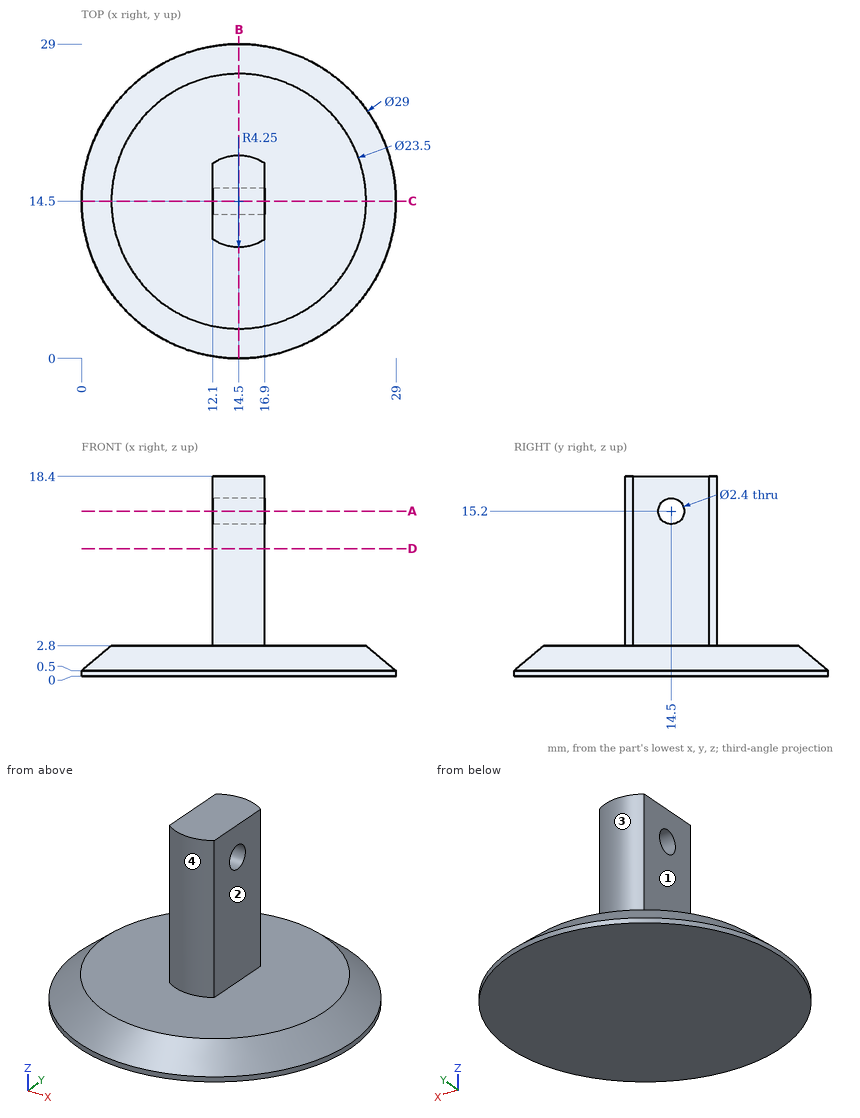
Study the drawing (mm; zero at the part's minimum x, y, z) and answer. A direction names the side the tool comes from. Round coordinates to 2 decimals unless told otherwise and drop trailing zeros. Loops run counter-clockwise (first coordinate to the right, second up) from the corner with the lowest first, then second, coordinate; pieces in that order, holes last. Notation, with made-up numbers: (-31, -1) -> (-6, -1) arc R7 ccw to (-6, 10) -> close; hole circle Ø11 at (18, 51). An arc over 180 degrees is marked (long way). Use one line per item in the form item = value.
1. A tool of negligible diameter and unlimited length cuts with its end or side. For the marked faces 1, 2, 3 and 4, from which of +Z, -Z, +X, -X, +Y, -Y can it reach the whole face along a straight path? Write none if from no direction.
Answer key:
face_1 = +Z, -X, +Y, -Y
face_2 = +Z, +X, +Y, -Y
face_3 = +Z, +Y
face_4 = +Z, -Y
2. Flat-ended cylindrical pins translate along their axes: pin 1 Ø3 at (x, z) = (11, 3.5) entering from +Y; pin 2 Ø6 at (y, z) = (16, 13) entering from +X; pin 3 Ø1.5 at (x, y) = (20, 3.5) entering from -Z; pin 4 Ø2 at (y, z) = (14.5, 15.2) entering from +X. Find the tip coordinate at first contact, or state that the pin passes through.
Answer key:
pin_1 = 26.76
pin_2 = 16.9
pin_3 = 0
pin_4 = through
3. The part is cut by section D-D on z = 11.75. Determine the outline of the cut face in (x, y).
Answer key:
outline = (12.1, 10.99) arc R4.25 ccw to (16.9, 10.99) -> (16.9, 18.01) arc R4.25 ccw to (12.1, 18.01) -> close
4. The part is cut by section A-A on z = 15.2. Determine the outline of the cut face in (x, y), and give its area (3 significant figures).
Answer key:
outline = (12.1, 10.99) arc R4.25 ccw to (16.9, 10.99) -> (16.9, 13.3) -> (12.1, 13.3) -> close; (12.1, 15.7) -> (16.9, 15.7) -> (16.9, 18.01) arc R4.25 ccw to (12.1, 18.01) -> close
area = 27.0 mm²
5. The part is cut by section B-B on x = 14.5. Determine the outline of the cut face in (y, z), and give its area (3 significant figures).
Answer key:
outline = (0, 0) -> (29, 0) -> (29, 0.5) -> (26.25, 2.8) -> (18.75, 2.8) -> (18.75, 18.4) -> (10.25, 18.4) -> (10.25, 2.8) -> (2.75, 2.8) -> (0, 0.5) -> close; hole circle Ø2.4 at (14.5, 15.2)
area = 203 mm²
6. The part is cut by section C-C on y = 14.5. Determine the outline of the cut face in (x, z), and give its area (3 significant figures).
Answer key:
outline = (0, 0) -> (29, 0) -> (29, 0.5) -> (26.25, 2.8) -> (16.9, 2.8) -> (16.9, 14) -> (12.1, 14) -> (12.1, 2.8) -> (2.75, 2.8) -> (0, 0.5) -> close; (12.1, 16.4) -> (16.9, 16.4) -> (16.9, 18.4) -> (12.1, 18.4) -> close
area = 138 mm²
7. Find the intervals of material crossed by probe 1 along Z at (x, y) = (15.5, 14.5); probe 2 along Z at (x, y) = (25, 11.5); probe 3 along X at (y, z) = (15, 11), in increasing order. Write a range as [from, to].
Answer key:
probe_1 = [0, 14], [16.4, 18.4]
probe_2 = [0, 2.8]
probe_3 = [12.1, 16.9]
